The figure shows three views and two pictorial views of one solid part (mm, origin at its lowest corner). Answer the questions. Round coordinates to 2 decimals unless told otherwise and drop trailing zeros. Order: outer loops, then holes, each group sorted by start corner. A loop starts at its lowest first (then second) coordinate and runs counter-clockwise, first axis right, second up. Notation, with made-up numbers: (-33, -13.75) - (3, -13.75) arc R16 ccw to (3, 2.25) - close; hole circle Ø8 at (86, 24.25). An arc over 180 degrees is marked (long way). Answer as a JSON object with one key per item and string values. Group by question number.
Q1. Given pin 1 Ø1.5 at (x, z) = (3.5, 3) entering from -Y; pin 2 Ø1.5 at (y, z) = (59, 3) entering from -X; pin 3 Ø1.5 at (y, z) = (10.5, 3.5) entering from +X, each flat-ended and moving along its own axis, determine where each tip first touches the part or whether it passes through.
Q2. A cutting plane is placed at C-C on z = 1.45. Determine the outline of the cut face in (x, y), and give its area (3 significant figures).
Q3. A cutting plane is placed at A-A on x = 11. Determine the outline of the cut face in (y, z).
Q4. A cutting plane is placed at D-D on x = 41. Determine the outline of the cut face in (y, z).
Q5. Consider line 1 (Y direction, x = 65, z = 1.45); line 2 (Y direction, x = 83, z = 1.8); line 3 (X direction, y = 49, z = 0.65). Determine where each line is inside the solid, lowest interval first.
Q6. A cutting plane is placed at B-B on y = 8.75. Determine the outline of the cut face in (x, z).
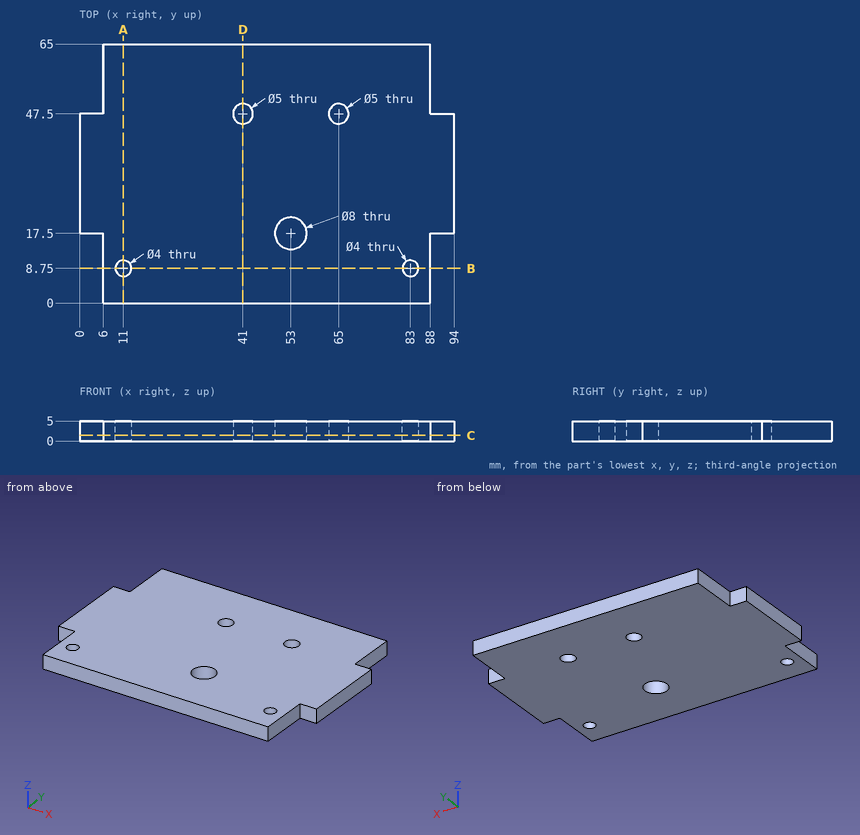
Result set:
{
 "1": {"pin 1": "stops at y = 17.5", "pin 2": "stops at x = 6", "pin 3": "stops at x = 88"},
 "2": {"outline": "(0, 17.5) - (6, 17.5) - (6, 0) - (88, 0) - (88, 17.5) - (94, 17.5) - (94, 47.5) - (88, 47.5) - (88, 65) - (6, 65) - (6, 47.5) - (0, 47.5) - close; hole circle Ø4 at (11, 8.75); hole circle Ø5 at (41, 47.5); hole circle Ø8 at (53, 17.5); hole circle Ø5 at (65, 47.5); hole circle Ø4 at (83, 8.75)", "area": "5,580 mm²"},
 "3": {"outline": "(0, 0) - (6.75, 0) - (6.75, 5) - (0, 5) - close; (10.75, 0) - (65, 0) - (65, 5) - (10.75, 5) - close"},
 "4": {"outline": "(0, 0) - (45, 0) - (45, 5) - (0, 5) - close; (50, 0) - (65, 0) - (65, 5) - (50, 5) - close"},
 "5": {"line 1": "y = 0 to 45, 50 to 65", "line 2": "y = 0 to 6.75, 10.75 to 65", "line 3": "x = 6 to 39, 43 to 63, 67 to 88"},
 "6": {"outline": "(6, 0) - (9, 0) - (9, 5) - (6, 5) - close; (13, 0) - (81, 0) - (81, 5) - (13, 5) - close; (85, 0) - (88, 0) - (88, 5) - (85, 5) - close"}
}
